Input: part model. Units: mm. Frame: model coordinates. Face numbers are marked on the shaded views. A direction names the side the tool comes from. Give positions to 0.01 mm unless a question says otherwise; leave off trailing zeros. Loops run counter-clockwise (first coordinate to the right, second up) from the corner with the lowest first, then second, coordinate; pieces in that order, holes last. Notation, with made-up numbers: M 10,4.25 L 46,4.25 A15 cw 46,21.25 Z; hole C 25,-21 d1. An arc over 180 degrees is marked long. Answer as a JSON object with one key per item and string values. Group by question number.
1) Draft query along Z for the marked faces 1, 2 and 3. Return one class per face: +Z half, -Z half, draft (parallel to the pull), parting line (faces both ways), or undercut.
2) Access query for the marked faces 4, 5 and 6. Directions: +Z, -Z, +X, -X, +Y, -Y. A direction counts if a zero-diameter tool reaches every point of the face in a straight line with its end or side. Return the directions, or none.
3) Section query D-D on y = 6.25. Return loops of the section in (x, z).
4) Section query A-A on x = 0. Return loops of the section in (y, z).
5) Ray query, L1, parallel to X at y = 4.75, z = 0; L2, parallel to Y at x = 1.85, z = -0.9; L3, parallel to Y at x = -1.2, z = 1.9. Return the intervals inside material, ascending.
6) Section query B-B on z = 0. Return loops of the section in (x, y), plus the area to 3 significant figures.
7) Section query C-C on y = 4. Return loops of the section in (x, z).
from build123d import *

# Parameters (mm, degrees)
SKETCH1_R           = 3
BOSS_EXTRUDE1_DEPTH = 1
CHAMFER1_SIZE       = 0.5
SKETCH2_R           = 2
BOSS_EXTRUDE2_DEPTH = 1
SKETCH3_R           = 2.5
BOSS_EXTRUDE3_DEPTH = 4
SKETCH4_R           = 2
BOSS_EXTRUDE4_DEPTH = 1
FILLET1_R           = 1
FILLET2_R           = 1
SKETCH5_R           = 1.5
CUT_EXTRUDE1_DEPTH  = 10


with BuildPart() as part:
    # Sketch1 → Boss-Extrude1 (new body)
    with BuildSketch(Plane(origin=(0, 0, 0), x_dir=(1, 0, 0), z_dir=(0, 1, 0))):
        with Locations(Location((0, 0, 0), (0, 0, 270))):
            Circle(SKETCH1_R)
    extrude(amount=BOSS_EXTRUDE1_DEPTH)

    # Chamfer1
    chamfer1_edges = [part.edges().sort_by_distance(p)[0] for p in [
        (0, 1, -3),
    ]]
    chamfer(chamfer1_edges, length=CHAMFER1_SIZE)

    # Sketch2 → Boss-Extrude2 (add)
    with BuildSketch(Plane(origin=(0, 1, 0), x_dir=(1, 0, 0), z_dir=(0, 1, 0))):
        with Locations(Location((0, 0, 0), (0, 0, 270))):
            Circle(SKETCH2_R)
    extrude(amount=BOSS_EXTRUDE2_DEPTH)

    # Sketch3 → Boss-Extrude3 (add)
    with BuildSketch(Plane(origin=(0, 2, 0), x_dir=(1, 0, 0), z_dir=(0, 1, 0))):
        with Locations(Location((0, 0, 0), (0, 0, 270))):
            Circle(SKETCH3_R)
    extrude(amount=BOSS_EXTRUDE3_DEPTH)

    # Sketch4 → Boss-Extrude4 (add)
    with BuildSketch(Plane(origin=(0, 6, 0), x_dir=(1, 0, 0), z_dir=(0, 1, 0))):
        with Locations(Location((0, 0, 0), (0, 0, 270))):
            Circle(SKETCH4_R)
    extrude(amount=BOSS_EXTRUDE4_DEPTH)

    # Fillet1
    # the kernel refuses this fillet: 1 mm, written as the material it takes off along each edge
    with BuildSketch(Plane(origin=(0, 6, 0), x_dir=(0, 0, 1), z_dir=(-1, 0, 0))) as fillet1_piece_1:
        with BuildLine():
            CenterArc((1.5, -0.866025404), FILLET1_R, 0, 60)
            Line((2, 0), (2.01, 0.017320508))
            ThreePointArc((2.01, 0.017320508), (2.25, 0.02), (2.5, 0.02))
            Line((2.5, 0.02), (2.52, 0))
            Line((2.52, 0), (2.52, -0.866025404))
            Line((2.52, -0.866025404), (2.5, -0.866025404))
        make_face()
    revolve(axis=Axis((0, 6, 0), (0, 1, 0)), mode=Mode.SUBTRACT)

    # Fillet2
    # the kernel refuses this fillet: 1 mm, written as the material it takes off along each edge
    with BuildSketch(Plane(origin=(0, 2, 0), x_dir=(0, 0, 1), z_dir=(-1, 0, 0))) as fillet2_piece_1:
        with BuildLine():
            CenterArc((1.5, 0.866025404), FILLET2_R, 300, 60)
            Line((2, 0), (2.01, -0.017320508))
            ThreePointArc((2.01, -0.017320508), (2.25, -0.02), (2.5, -0.02))
            Line((2.5, -0.02), (2.52, 0))
            Line((2.52, 0), (2.52, 0.866025404))
            Line((2.52, 0.866025404), (2.5, 0.866025404))
        make_face()
    revolve(axis=Axis((0, 2, 0), (0, 1, 0)), mode=Mode.SUBTRACT)

    # Sketch5 → Cut-Extrude1 (cut)
    with BuildSketch(Plane.XZ):
        with Locations(Location((0, 0, 0), (0, 0, 270))):
            Circle(SKETCH5_R)
    extrude(amount=-CUT_EXTRUDE1_DEPTH, mode=Mode.SUBTRACT)


solid = part.part
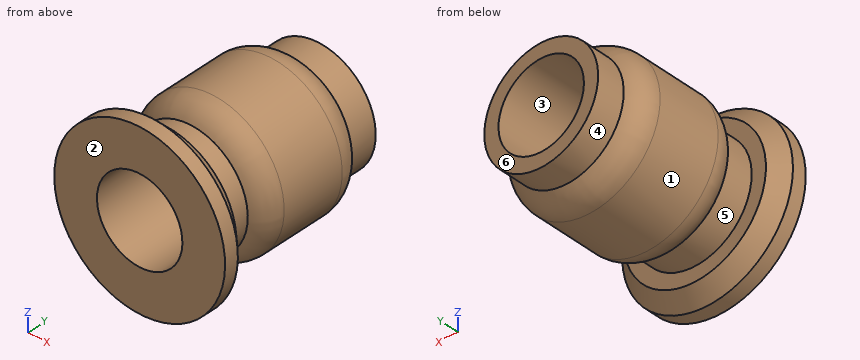
Output:
{
 "1": {"face 1": "parting line", "face 2": "draft", "face 3": "undercut"},
 "2": {"face 4": "+Y", "face 5": "none", "face 6": "+Z, -Z, +X, -X, +Y"},
 "3": {"outline": "C 0,0 d4; hole C 0,0 d3"},
 "4": {"outline": "M 0,-3 L 0.5,-3 L 1,-2.5 L 1,-2 L 2,-2 A1 ccw 2.87,-2.5 L 5.13,-2.5 A1 ccw 6,-2 L 7,-2 L 7,-1.5 L 0,-1.5 Z; M 0,1.5 L 7,1.5 L 7,2 L 6,2 A1 ccw 5.13,2.5 L 2.87,2.5 A1 ccw 2,2 L 1,2 L 1,2.5 L 0.5,3 L 0,3 Z"},
 "5": {"L1": "x = -2.5 to -1.5, 1.5 to 2.5", "L2": "y = 0 to 1, 2.04 to 5.96", "L3": "y = 0 to 1, 2.2 to 5.8"},
 "6": {"outline": "M -3,0 L -1.5,0 L -1.5,7 L -2,7 L -2,6 A1 ccw -2.5,5.13 L -2.5,2.87 A1 ccw -2,2 L -2,1 L -2.5,1 L -3,0.5 Z; M 1.5,0 L 3,0 L 3,0.5 L 2.5,1 L 2,1 L 2,2 A1 ccw 2.5,2.87 L 2.5,5.13 A1 ccw 2,6 L 2,7 L 1.5,7 Z", "area": "12.2 mm^2"},
 "7": {"outline": "C 0,0 d5; hole C 0,0 d3"}
}
